```python
from build123d import *

# Parameters (mm, degrees)
F0_W     = 38.1
F0_H     = 88.9
F1_DEPTH = 889
F3_DEPTH = 25.4
F5_DEPTH = 25.4


with BuildPart() as f1:
    # F0 (on Front) → F1 (new body)
    with BuildSketch(Plane.XZ):
        Rectangle(F0_W, F0_H)
    extrude(amount=F1_DEPTH)

    # F2 (on Right) → F3 (cut, symmetric)
    with BuildSketch(Plane.YZ):
        Polygon((-889, -44.45), (-865.124, 44.45), (-889, 44.45), align=None)
    extrude(amount=F3_DEPTH, both=True, mode=Mode.SUBTRACT)

    # F4 (on Right) → F5 (cut, symmetric)
    with BuildSketch(Plane.YZ):
        Polygon((0, -44.45), (0, 44.45), (-23.876, -44.45), align=None)
    extrude(amount=F5_DEPTH, both=True, mode=Mode.SUBTRACT)


solid = f1.part
```
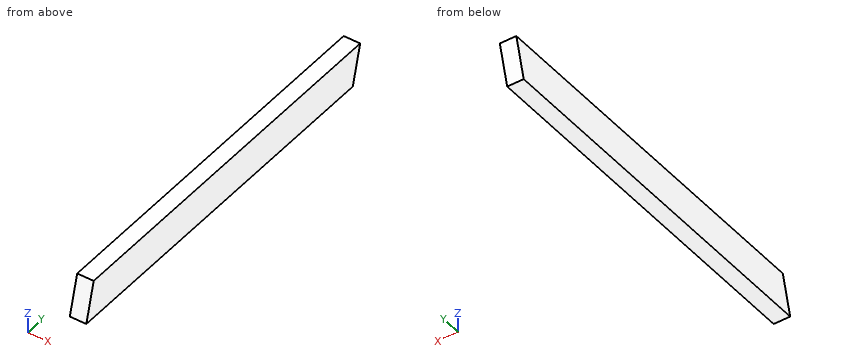
Can you work these out from the model? Positions are in its coordinate system, mm. Coordinates: 2 decimals unless noted, no trailing zeros. Loops run counter-clockwise (first coordinate to the right, second up) from the corner with the lowest first, then second, coordinate; pieces in that order, holes last. Notation, with made-up numbers: M 69,48.25 L 82,48.25 A18 ccw 82,69.25 Z; hole C 49.5,57.5 d3. An arc over 180 degrees is marked long. Put each result on its own line as item: value. Start each with the question number.
(1) Imagine slicing it at A-A on x = -6. List the corners of the cut face in (y, z) for me.
(2) I need wall thicknesses on probe 1 along Y at (x, z) = (2.5, 27.5); probe 2 along Y at (x, z) = (5, 2). Which ranges of each line are inside material? Lowest first, please.
(3) Will these pins go through, and if not, where does the flat tip stop? pin 1 Ø3 at (x, z) = (-0.5, -20.5) entering from -Y; pin 2 Ø1.5 at (x, z) = (10, 19.5) entering from +Y; pin 3 Ø12 at (x, z) = (12.5, -20) entering from +Y.
(4) Imagine slicing it at B-B on z = -30. List the corners of the cut face in (x, y) for me.
Worked answers:
1. outline: M -889,-44.45 L -23.88,-44.45 L 0,44.45 L -865.12,44.45 Z
2. probe 1: y = -869.68 to -4.55
2. probe 2: y = -876.52 to -11.4
3. pin 1: stops at y = -882.97
3. pin 2: stops at y = -6.5
3. pin 3: stops at y = -15.7
4. outline: M -19.05,-885.12 L 19.05,-885.12 L 19.05,-20 L -19.05,-20 Z
